Read the model definition and answer for the solid it produces. Units are mm, in the model's axes. Face numbers are marked on the shaded views. A direction names the side the tool comes from. Round coordinates to 2 decimals unless told otherwise and drop trailing zeros. Order: outer loops, then holes, each group sorted by start corner. A loop starts at its lowest first (then second) coordinate and runs counter-clockwise, first axis right, second up.
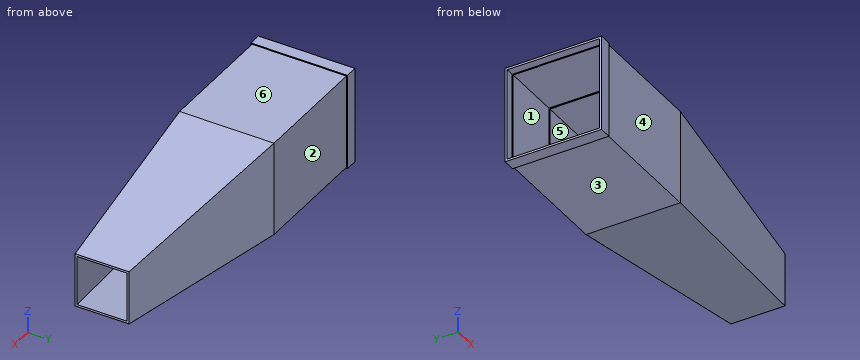
from build123d import *

# Parameters (mm, degrees)
SKETCH1_W               = 232.5
SKETCH1_H               = 232.5
SKETCH1_W_2             = 222.5
SKETCH1_H_2             = 222.5
BOSS_EXTRUDE1_DEPTH     = 30
SKETCH3_W               = 227.5
SKETCH3_H               = 227.5
SKETCH3_W_2             = 217.5
SKETCH3_H_2             = 217.5
BOSS_EXTRUDE2_DEPTH     = 300
CUT_EXTRUDE1_DEPTH      = 2
CUT_EXTRUDE1_DEPTH_BACK = 2
SKETCH8_W               = 222.5
SKETCH8_H               = 222.5
SKETCH8_W_2             = 217.5
SKETCH8_H_2             = 217.5


with BuildPart() as part:
    # Sketch1 → Boss-Extrude1 (new body)
    with BuildSketch(Plane(origin=(0, 0, 0), x_dir=(0, 0, -1), z_dir=(1, 0, 0))):
        Rectangle(SKETCH1_W, SKETCH1_H)
        Rectangle(SKETCH1_W_2, SKETCH1_H_2, mode=Mode.SUBTRACT)
    extrude(amount=BOSS_EXTRUDE1_DEPTH)

    # Sketch3 → Boss-Extrude2 (add)
    with BuildSketch(Plane(origin=(20, 0, 0), x_dir=(0, 0, -1), z_dir=(1, 0, 0))):
        Rectangle(SKETCH3_W, SKETCH3_H)
        Rectangle(SKETCH3_W_2, SKETCH3_H_2, mode=Mode.SUBTRACT)
    extrude(amount=BOSS_EXTRUDE2_DEPTH)

    # Sketch5 → Loft2 section 0
    with BuildSketch(Plane(origin=(320, 0, 0), x_dir=(0, 0, -1), z_dir=(1, 0, 0))):
        with BuildLine():
            Line((-113.75, 113.75), (113.75, 113.75))
            Line((113.75, 113.75), (113.75, -113.75))
            Line((113.75, -113.75), (-113.75, -113.75))
            Line((-113.75, -113.75), (-113.75, 113.75))
        make_face()
    # Sketch4 → Loft2 section 1
    with BuildSketch(Plane(origin=(820, 0, 0), x_dir=(0, 0, -1), z_dir=(1, 0, 0))):
        with BuildLine():
            Line((-65, 65), (65, 65))
            Line((65, 65), (65, -65))
            Line((65, -65), (-65, -65))
            Line((-65, -65), (-65, 65))
        make_face()
    loft()

    # Sketch5<5> → Cut-Loft2 section 0
    with BuildSketch(Plane(origin=(320, 0, 0), x_dir=(0, 0, -1), z_dir=(1, 0, 0))):
        with BuildLine():
            Line((-108.75, 108.75), (108.75, 108.75))
            Line((108.75, 108.75), (108.75, -108.75))
            Line((108.75, -108.75), (-108.75, -108.75))
            Line((-108.75, -108.75), (-108.75, 108.75))
        make_face()
    # Sketch4<7> → Cut-Loft2 section 1
    with BuildSketch(Plane(origin=(820, 0, 0), x_dir=(0, 0, -1), z_dir=(1, 0, 0))):
        with BuildLine():
            Line((-60, 60), (60, 60))
            Line((60, 60), (60, -60))
            Line((60, -60), (-60, -60))
            Line((-60, -60), (-60, 60))
        make_face()
    loft(mode=Mode.SUBTRACT)

    # Sketch8 → Cut-Extrude1 (cut, two sides: drawn at the far end of the back side and taken through both)
    with BuildSketch(Plane(origin=(165, 0, 0), x_dir=(0, 0, -1), z_dir=(1, 0, 0)).offset(-CUT_EXTRUDE1_DEPTH_BACK)):
        Rectangle(SKETCH8_W, SKETCH8_H)
        Rectangle(SKETCH8_W_2, SKETCH8_H_2, mode=Mode.SUBTRACT)
    extrude(amount=CUT_EXTRUDE1_DEPTH + CUT_EXTRUDE1_DEPTH_BACK, mode=Mode.SUBTRACT)


solid = part.part
Q1. For a pull along Y with two mould halves and no side action, classify the marked faces 1, 2 and 3 as released by +Y, released by -Y, zero draft, split by the parting line, or undercut.
Outcome:
face 1: undercut
face 2: released by +Y
face 3: zero draft
Q2. A cutting plane is placed at A-A, the plane x = 116. Give the vertices of the cut face in (y, z), plus the area to 3 significant figures.
Outcome:
outline: (-113.75, -113.75) - (113.75, -113.75) - (113.75, 113.75) - (-113.75, 113.75) - close; hole (-108.75, -108.75) - (108.75, -108.75) - (108.75, 108.75) - (-108.75, 108.75) - close
area: 4,450 mm2
Q3. Flat-ended cylindrical pins translate along their axes: pin 1 (3 mm diameter, centred on x = 164, z = 41, fed in from -Y); pin 2 (3 mm diameter, centred on x = 378.5, z = -87.5, fed in from -Y); pin 3 (10 mm diameter, centred on x = 180.5, y = -79, fed in from +Z). Find the tip coordinate at first contact, or state that the pin passes through.
Outcome:
pin 1: stops at y = -113.75
pin 2: stops at y = -108.19
pin 3: stops at z = 113.75
Q4. Straight lines are drawn through the part: probe 1 along Y at (x, z) = (95.5, -56.5); probe 2 along Z at (x, y) = (165.5, 11.5). For each, find the intervals that lie inside material, in ascending order.
Outcome:
probe 1: y = -113.75 to -108.75, 108.75 to 113.75
probe 2: z = -113.75 to -111.25, 111.25 to 113.75
Q5. For the marked faces 4, 5 and 6, determine the directions among +Z, -Z, +X, -X, +Y, -Y from which every point of the face is accessible in a straight line to the end or side of a thin tool.
Outcome:
face 4: +Z, -Z, +X, -Y
face 5: -X
face 6: +Z, +X, +Y, -Y
